For this review, use the dimensioned drawing (mm, ordinates from the lowest corner) and the shaded views. Coordinates: 2 decimals unless noted, no trailing zeros. Loops run counter-clockwise (first coordinate to the right, second up) from the corner with the lowest first, then second, coordinate; pieces in that order, holes last. Notation, with made-up numbers: (-22, -34) - (14, -34) arc R3 ccw to (14, -30) - close; hole circle Ø3 at (-11, 64.5). An arc over 180 degrees is marked (long way). Answer in a Markdown table with one row per item. Add a question column.
(1) We need section A-A on y = 29. Write out the cut boundary in (x, z).
(2) We need section D-D on y = 49. Write out the cut boundary in (x, z), plus the area to 3 significant figures.
(3) We need section C-C on z = 2.4. Give the number of separate pieces and of enclosed holes in the cut face, plus the area to 3 significant figures.
(4) For line 1 along Y through (x, z) = (69, 2); line 2 along X through (y, z) = (50.5, 2.2); line 3 along X through (y, z) = (29.5, 2.1), list the stretches that pass through material, from the lowest coordinate up.
(5) We need section B-B on x = 9. Write out the cut boundary in (y, z), plus the area to 3 significant figures.
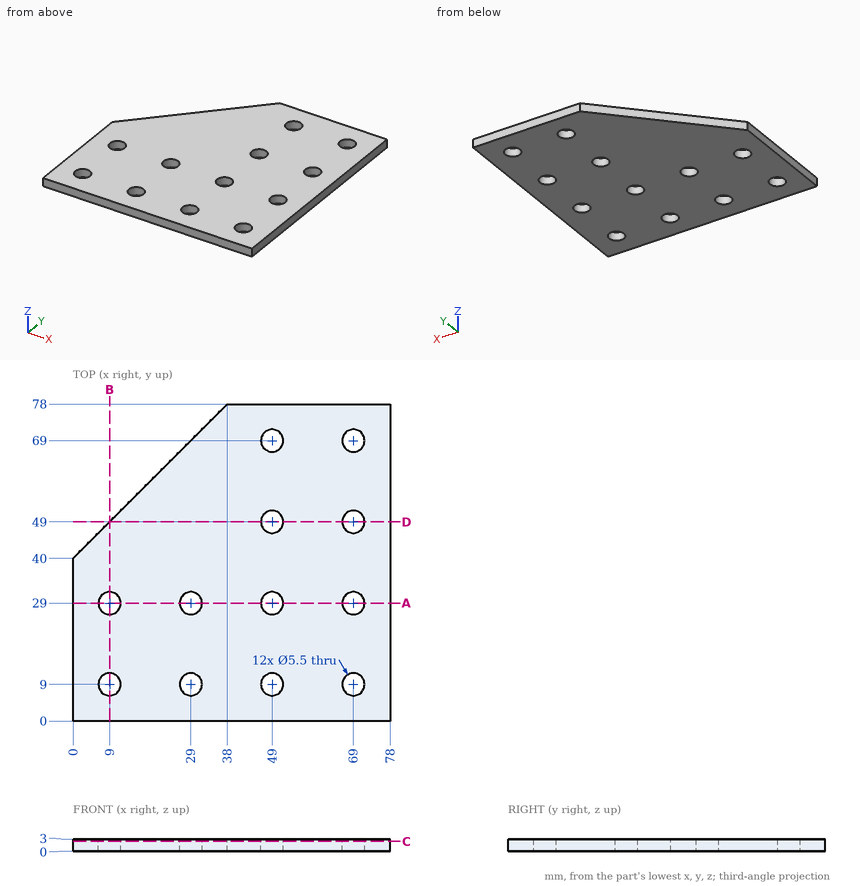
Outcome:
| question | item | result |
|---|---|---|
| 1 | outline | (0, 0) - (6.25, 0) - (6.25, 3) - (0, 3) - close; (11.75, 0) - (26.25, 0) - (26.25, 3) - (11.75, 3) - close; (31.75, 0) - (46.25, 0) - (46.25, 3) - (31.75, 3) - close; (51.75, 0) - (66.25, 0) - (66.25, 3) - (51.75, 3) - close; (71.75, 0) - (78, 0) - (78, 3) - (71.75, 3) - close |
| 2 | outline | (9, 0) - (46.25, 0) - (46.25, 3) - (9, 3) - close; (51.75, 0) - (66.25, 0) - (66.25, 3) - (51.75, 3) - close; (71.75, 0) - (78, 0) - (78, 3) - (71.75, 3) - close |
| 2 | area | 174 mm² |
| 3 | separate pieces | 1 |
| 3 | enclosed holes | 12 |
| 3 | area | 5,080 mm² |
| 4 | line 1 | 0 to 6.25, 11.75 to 26.25, 31.75 to 46.25, 51.75 to 66.25, 71.75 to 78 |
| 4 | line 2 | 10.5 to 46.7, 51.3 to 66.7, 71.3 to 78 |
| 4 | line 3 | 0 to 6.3, 11.7 to 26.3, 31.7 to 46.3, 51.7 to 66.3, 71.7 to 78 |
| 5 | outline | (0, 0) - (6.25, 0) - (6.25, 3) - (0, 3) - close; (11.75, 0) - (26.25, 0) - (26.25, 3) - (11.75, 3) - close; (31.75, 0) - (49, 0) - (49, 3) - (31.75, 3) - close |
| 5 | area | 114 mm² |
